from build123d import *

# Parameters (mm, degrees)
SKETCH1_W             = 50.8
SKETCH1_H             = 76.2
BOSS_EXTRUDE1_DEPTH   = 100
SKETCH2_W             = 46.8
SKETCH2_H             = 72.2
CUT_EXTRUDE1_DEPTH    = 110.985317202
FILLET2_R             = 2
CORTAR_EXTRUIR2_DEPTH = 10
CROQUIS4_R            = 2.5
CORTAR_EXTRUIR5_DEPTH = 10
CROQUIS6_R            = 2.5
CORTAR_EXTRUIR6_DEPTH = 10
CROQUIS7_R            = 2.5
CORTAR_EXTRUIR7_DEPTH = 10


with BuildPart() as part:
    # Sketch1 → Boss-Extrude1 (new body)
    with BuildSketch(Plane(origin=(0, 0, 0), x_dir=(0, 0, -1), z_dir=(1, 0, 0))):
        Rectangle(SKETCH1_W, SKETCH1_H)
    extrude(amount=-BOSS_EXTRUDE1_DEPTH)

    # Sketch2 → Cut-Extrude1 (cut, through all)
    with BuildSketch(Plane(origin=(0, 0, 0), x_dir=(0, 0, -1), z_dir=(1, 0, 0))):
        Rectangle(SKETCH2_W, SKETCH2_H)
    extrude(amount=-CUT_EXTRUDE1_DEPTH, mode=Mode.SUBTRACT)

    # Fillet2
    fillet2_edges = [part.edges().sort_by_distance(p)[0] for p in [
        (-50, -36.1, 23.4),
        (-50, 36.1, 23.4),
        (-50, 36.1, -23.4),
        (-50, -36.1, -23.4),
        (-50, 38.1, 25.4),
        (-50, 38.1, -25.4),
        (-50, -38.1, -25.4),
        (-50, -38.1, 25.4),
    ]]
    fillet(fillet2_edges, radius=FILLET2_R)

    # Croquis2 → Cortar-Extruir2 (cut)
    with BuildSketch(Plane.XY.offset(25.4)):
        with BuildLine():
            ThreePointArc((-27, 26.5), (-30, 29.5), (-33, 26.5))
            Line((-33, 26.5), (-30, 26.5))
            Line((-30, 26.5), (-30, 23.5))
            ThreePointArc((-30, 23.5), (-27.878679656, 24.378679656), (-27, 26.5))
        make_face()
        with BuildLine():
            Line((-30, 26.5), (-33, 26.5))
            ThreePointArc((-33, 26.5), (-32.121320344, 24.378679656), (-30, 23.5))
            Line((-30, 23.5), (-30, 26.5))
        make_face()
        with BuildLine():
            ThreePointArc((-70, 23.5), (-67.878679656, 24.378679656), (-67, 26.5))
            Line((-67, 26.5), (-70, 26.5))
            Line((-70, 26.5), (-70, 23.5))
        make_face()
        with BuildLine():
            Line((-70, 26.5), (-67, 26.5))
            ThreePointArc((-67, 26.5), (-72.121320344, 28.621320344), (-70, 23.5))
            Line((-70, 23.5), (-70, 26.5))
        make_face()
        with BuildLine():
            ThreePointArc((-67, -26.5), (-67.878679656, -24.378679656), (-70, -23.5))
            Line((-70, -23.5), (-70, -26.5))
            Line((-70, -26.5), (-67, -26.5))
        make_face()
        with BuildLine():
            Line((-70, -26.5), (-70, -23.5))
            ThreePointArc((-70, -23.5), (-72.121320344, -28.621320344), (-67, -26.5))
            Line((-67, -26.5), (-70, -26.5))
        make_face()
        with BuildLine():
            ThreePointArc((-27, -26.5), (-27.878679656, -24.378679656), (-30, -23.5))
            Line((-30, -23.5), (-30, -26.5))
            Line((-30, -26.5), (-33, -26.5))
            ThreePointArc((-33, -26.5), (-30, -29.5), (-27, -26.5))
        make_face()
        with BuildLine():
            Line((-30, -26.5), (-30, -23.5))
            ThreePointArc((-30, -23.5), (-32.121320344, -24.378679656), (-33, -26.5))
            Line((-33, -26.5), (-30, -26.5))
        make_face()
    extrude(amount=-CORTAR_EXTRUIR2_DEPTH, mode=Mode.SUBTRACT)

    # Croquis4 → Cortar-Extruir5 (cut)
    with BuildSketch(Plane(origin=(0, 0, -25.4), x_dir=(-1, 0, 0), z_dir=(0, 0, -1))):
        with Locations(Location((90, 23.1, 0), (0, 0, 90))):
            Circle(CROQUIS4_R)
        with Locations(Location((59.2, 23.1, 0), (0, 0, 90))):
            Circle(CROQUIS4_R)
        with Locations(Location((59.2, -23.1, 0), (0, 0, 90))):
            Circle(CROQUIS4_R)
        with Locations(Location((90, -23.1, 0), (0, 0, 90))):
            Circle(CROQUIS4_R)
        with Locations(Location((74.6, 0, 0), (0, 0, 90))):
            Circle(CROQUIS4_R)
    extrude(amount=-CORTAR_EXTRUIR5_DEPTH, mode=Mode.SUBTRACT)

    # Croquis6 → Cortar-Extruir6 (cut)
    with BuildSketch(Plane(origin=(0, 0, -25.4), x_dir=(-1, 0, 0), z_dir=(0, 0, -1))):
        with Locations(Location((17.2, 20, 0), (0, 0, 90))):
            Circle(CROQUIS6_R)
        with Locations(Location((17.2, -20, 0), (0, 0, 90))):
            Circle(CROQUIS6_R)
        with Locations(Location((41.2, -20, 0), (0, 0, 90))):
            Circle(CROQUIS6_R)
        with Locations(Location((41.2, 20, 0), (0, 0, 90))):
            Circle(CROQUIS6_R)
    extrude(amount=-CORTAR_EXTRUIR6_DEPTH, mode=Mode.SUBTRACT)

    # Croquis7 → Cortar-Extruir7 (cut)
    with BuildSketch(Plane(origin=(0, 38.1, 0), x_dir=(1, 0, 0), z_dir=(0, 1, 0))):
        with Locations(Location((-80, -0.4, 0), (0, 0, 270))):
            Circle(CROQUIS7_R)
        with Locations(Location((-20, -0.4, 0), (0, 0, 270))):
            Circle(CROQUIS7_R)
    extrude(amount=-CORTAR_EXTRUIR7_DEPTH, mode=Mode.SUBTRACT)


solid = part.part
Work out the finished part from the listing and answer in its coordinate system (mm). A direction names the side the tool comes from. Coordinates: 2 decimals unless noted, no trailing zeros. Write each loop counter-clockwise with the first axis right and the second up, starting at its lowest first coordinate (ties: lowest second). Pieces come first, ordered by that corner, then holes. Notation, with made-up numbers: M 47,69.25 L 86,69.25 A15 cw 86,74.25 Z; hole C -2,85.25 d1. An arc over 180 degrees is marked long. Use one line per item in the form item = value. Start each with the question number.
1. The mould has two halves that part along X. Classify faces 6 (the face through (-77.04, -0.54, -24.41)), 7 (the face through (-100, 0, 25)), 8 (the face through (-49, -38.1, 0)): released by +X, released by -X, zero draft, split by the parting line, or undercut.
2. The part is cut by section C-C (z = 8). Give the vertices of the cut face in (x, y).
3. The part is cut by section B-B (y = -6.5). Give the vertices of the cut face in (x, z).
4. A tool of negligible diameter and unlimited length cuts with its end or side. For faces 1 (the face through (-42.7, 18, -24.4)), 2 (the face through (-49, 0, 23.4)), 3 (the face through (-17.52, 37.11, 0.07)), 4 (the face through (-49, 38.1, 0)), 5 (the face through (0, 0, 25)), from which of +Z, -Z, +X, -X, +Y, -Y can it reach the whole face along a straight path? Write none if from no direction.
5. Straight lines are drawn through the part: probe 1 along X at (y, z) = (36.75, 0.4); probe 2 along X at (y, z) = (-20, -24.7); probe 3 along Z at (x, y) = (-87, 13.5). For each, find the intervals that lie inside material, in ascending order. Write a range as from..to.
6. The part is cut by section D-D (z = 0.5). Give the vertices of the cut face in (x, y), plus the area to 3 significant figures.
7. The part is cut by section A-A (x = -55). Give the vertices of the cut face in (y, z), plus the area to 3 significant figures.
8. This flat-tipped pin is pushed along its axis until it touches: P1, Ø3, axis at x = -74.6, y = 0, coming from the -Z side. Where does it stop, or does it pass through?
Evaluation:
q1.face_6 = undercut
q1.face_7 = released by -X
q1.face_8 = zero draft
q2.outline = M -100,-38.1 L 0,-38.1 L 0,-36.1 L -100,-36.1 Z; M -100,36.1 L 0,36.1 L 0,38.1 L -100,38.1 Z
q3.outline = M -100,-25.4 L 0,-25.4 L 0,-23.4 L -100,-23.4 Z; M -100,23.4 L 0,23.4 L 0,25.4 L -100,25.4 Z
q4.face_1 = -Z
q4.face_2 = +X, -X
q4.face_3 = +Y
q4.face_4 = +Z, -Z, +X, -X, +Y
q4.face_5 = +Z, -Z, +X, +Y, -Y
q5.probe_1 = -100..-82.5, -77.5..-22.5, -17.5..0
q5.probe_2 = -100..-43.7, -38.7..-19.7, -14.7..0
q5.probe_3 = -25.4..-23.4, 23.4..25.4
q6.outline = M -100,-38.1 L 0,-38.1 L 0,-36.1 L -100,-36.1 Z; M -100,36.1 L -82.5,36.1 L -82.5,38.1 L -100,38.1 Z; M -77.5,36.1 L -22.5,36.1 L -22.5,38.1 L -77.5,38.1 Z; M -17.5,36.1 L 0,36.1 L 0,38.1 L -17.5,38.1 Z
q6.area = 380 mm^2
q7.outline = M -38.1,-23.4 A2 ccw -36.1,-25.4 L 36.1,-25.4 A2 ccw 38.1,-23.4 L 38.1,23.4 A2 ccw 36.1,25.4 L -36.1,25.4 A2 ccw -38.1,23.4 Z; hole M -36.1,-21.4 A2 ccw -34.1,-23.4 L 34.1,-23.4 A2 ccw 36.1,-21.4 L 36.1,21.4 A2 ccw 34.1,23.4 L -34.1,23.4 A2 ccw -36.1,21.4 Z
q7.area = 492 mm^2
q8.P1 = 23.4
